Can you work these out from the model? Positions are in its coordinate system, mm. A direction names the side the tool comes from. Coordinates: 2 decimals unless noted, no trailing zeros. Order: outer loops, then holes, each group sorted by start corner. A loop starts at its lowest first (then second) coordinate and runs counter-clockwise, first axis right, second up. Notation, with made-up numbers: (54.5, 28) -> (83.5, 28) arc R33 ccw to (83.5, 60) -> close; hole circle Ø10 at (81, 74). An arc over 180 degrees is marked (long way). Answer in a Markdown table with one row per item.
```python
from build123d import *

# Parameters (mm, degrees)
SKETCH1_W           = 42.3
SKETCH1_H           = 42.3
SKETCH1_R           = 1.75
SKETCH1_R_2         = 11.5
BOSS_EXTRUDE1_DEPTH = 8
BOSS_EXTRUDE2_START = -10
BOSS_EXTRUDE2_DEPTH = 22.3
SKETCH4_R           = 2.75
CUT_EXTRUDE1_DEPTH  = 62.713839627
SKETCH5_R           = 3.75
SKETCH5_R_2         = 1.75
BOSS_EXTRUDE3_DEPTH = 4.3
SKETCH7_R           = 4.25
CUT_EXTRUDE2_DEPTH  = 2
CUT_EXTRUDE3_START  = -2
SKETCH8_R           = 4.25
CUT_EXTRUDE3_DEPTH  = 2


with BuildPart() as part:
    # Sketch1 → Boss-Extrude1 (new body)
    with BuildSketch(Plane(origin=(0, 0, 0), x_dir=(1, 0, 0), z_dir=(0, 1, 0))):
        Rectangle(SKETCH1_W, SKETCH1_H)
        with Locations(Location((-15.5, 15.5, 0), (0, 0, 270))):
            Circle(SKETCH1_R, mode=Mode.SUBTRACT)
        with Locations(Location((15.5, 15.5, 0), (0, 0, 90))):
            Circle(SKETCH1_R, mode=Mode.SUBTRACT)
        with Locations(Location((15.5, -15.5, 0), (0, 0, 270))):
            Circle(SKETCH1_R, mode=Mode.SUBTRACT)
        with Locations(Location((-15.5, -15.5, 0), (0, 0, 90))):
            Circle(SKETCH1_R, mode=Mode.SUBTRACT)
        with Locations(Location((0, 0, 0), (0, 0, 270))):
            Circle(SKETCH1_R_2, mode=Mode.SUBTRACT)
    extrude(amount=BOSS_EXTRUDE1_DEPTH)

    # Sketch3 → Boss-Extrude2 (add)
    with BuildSketch(Plane.XY.offset(21.15).offset(BOSS_EXTRUDE2_START)):
        Polygon((-21.15, 8), (-21.15, 18.080453059), (-15.4, 25.004144271), (-15.4, 45.004144271), (-10.4, 45.004144271), (-10.4, 23.198658368), (-16.15, 16.274967156), (-16.15, 8), align=None)
        Polygon((16.15, 16.274967156), (16.15, 8), (21.15, 8), (21.15, 18.080453059), (15.4, 25.004144271), (15.4, 45.004144271), (10.4, 45.004144271), (10.4, 23.198658368), align=None)
    extrude(amount=-BOSS_EXTRUDE2_DEPTH)

    # Sketch4 → Cut-Extrude1 (cut, through all)
    with BuildSketch(Plane.ZY.offset(15.4)):
        with Locations(Location((-6.081010951, 35.004144271, 0), (0, 0, 270))):
            Circle(SKETCH4_R)
        with Locations(Location((6.081010951, 35.004144271, 0), (0, 0, 270))):
            Circle(SKETCH4_R)
    extrude(amount=-CUT_EXTRUDE1_DEPTH, mode=Mode.SUBTRACT)

    # Sketch5 → Boss-Extrude3 (add)
    # profile 1 of 4: a face of its own
    with BuildSketch(Plane(origin=(0, 8, 0), x_dir=(1, 0, 0), z_dir=(0, 1, 0))):
        with Locations(Location((-15.5, 15.5, 0), (0, 0, 90))):
            Circle(SKETCH5_R)
        with Locations(Location((-15.5, 15.5, 0), (0, 0, 270))):
            Circle(SKETCH5_R_2, mode=Mode.SUBTRACT)
    # profile 2 of 4: a face of its own
    with BuildSketch(Plane(origin=(0, 8, 0), x_dir=(1, 0, 0), z_dir=(0, 1, 0))):
        with Locations(Location((15.5, 15.5, 0), (0, 0, 90))):
            Circle(SKETCH5_R)
        with Locations(Location((15.5, 15.5, 0), (0, 0, 90))):
            Circle(SKETCH5_R_2, mode=Mode.SUBTRACT)
    # profile 3 of 4: a face of its own
    with BuildSketch(Plane(origin=(0, 8, 0), x_dir=(1, 0, 0), z_dir=(0, 1, 0))):
        with Locations(Location((15.5, -15.5, 0), (0, 0, 90))):
            Circle(SKETCH5_R)
        with Locations(Location((15.5, -15.5, 0), (0, 0, 270))):
            Circle(SKETCH5_R_2, mode=Mode.SUBTRACT)
    # profile 4 of 4: a face of its own
    with BuildSketch(Plane(origin=(0, 8, 0), x_dir=(1, 0, 0), z_dir=(0, 1, 0))):
        with Locations(Location((-15.5, -15.5, 0), (0, 0, 90))):
            Circle(SKETCH5_R)
        with Locations(Location((-15.5, -15.5, 0), (0, 0, 90))):
            Circle(SKETCH5_R_2, mode=Mode.SUBTRACT)
    extrude(amount=BOSS_EXTRUDE3_DEPTH)

    # Sketch7 → Cut-Extrude2 (cut)
    with BuildSketch(Plane.ZY.offset(15.4)):
        with Locations((-6.081010951, 35.004144271)):
            Circle(SKETCH7_R)
        with Locations((6.081010951, 35.004144271)):
            Circle(SKETCH7_R)
    extrude(amount=-CUT_EXTRUDE2_DEPTH, mode=Mode.SUBTRACT)

    # Sketch8 → Cut-Extrude3 (cut)
    with BuildSketch(Plane(origin=(15.4, 0, 0), x_dir=(0, 0, -1), z_dir=(1, 0, 0)).offset(CUT_EXTRUDE3_START)):
        with Locations(Location((-6.081010951, 35.004144271, 0), (0, 0, 180))):
            Circle(SKETCH8_R)
        with Locations(Location((6.081010951, 35.004144271, 0), (0, 0, 180))):
            Circle(SKETCH8_R)
    extrude(amount=CUT_EXTRUDE3_DEPTH, mode=Mode.SUBTRACT)


solid = part.part
```
(1) We'd pull the mould along Z, two halves only. Please class faces 6 (the flat face through (0, 4, -21.15)), 7 (the cylindrical face through (-11.921, 32.464, 5.028)), 8 (the flat face through (13.23, 19.79, 0.16)): +Z half, -Z half, draft (parallel to the pull), parting line (faces both ways), or undercut.
Response values:
| item | result |
|---|---|
| face 6 | -Z half |
| face 7 | undercut |
| face 8 | draft |
(2) On a 3-axis mill with a long thin cutter (end or side, diameter ignored), from which of +Z, -Z, +X, -X, +Y, -Y can I reach the whole of each face in a straight line? I mean faces 1 (the cylindrical face through (-14.414, 30.855, 5.16)), 2 (the flat face through (-10, 8, -10)), 3 (the cylindrical face through (9.7, 3.94, 6.18)), 4 (the cylindrical face through (14.39, 30.79, -6.63)), 5 (the flat face through (13, 45.004, 0)). Say none if no direction works.
Response values:
| item | result |
|---|---|
| face 1 | -X |
| face 2 | none |
| face 3 | -Y |
| face 4 | +X |
| face 5 | +Z, -Z, +X, -X, +Y |
(3) Will these pins go through, and if not, where does the flat tip stop? pin 1 Ø5 at (y, z) = (12, 16.5) entering from -X; pin 2 Ø3.5 at (y, z) = (35, -6.08) entering from -X; pin 3 Ø8 at (x, y) = (-7.5, 22.5) entering from -Z; pin 4 Ø6 at (y, z) = (38, -0.5) entering from +X.
Response values:
| item | result |
|---|---|
| pin 1 | x = -19.25 |
| pin 2 | through |
| pin 3 | z = -11.15 |
| pin 4 | x = 15.4 |
(4) I need wall thicknesses on line 1 (X direction, y = 6, z = -15.5); line 2 (Z direction, x = 14, y = 34); line 3 (Y direction, x = 15, z = 5). Which ranges of each line are inside material? Lowest first, please. Write a range as [from, to].
Response values:
| item | result |
|---|---|
| line 1 | [-21.15, -17.25], [-13.75, 13.75], [17.25, 21.15] |
| line 2 | [-11.15, -10.21], [-1.95, 1.95], [10.21, 11.15] |
| line 3 | [0, 8], [17.66, 30.89], [39.11, 45] |
(5) Suppose I cut it at A-A (x = 0). Please give me the cut outline in (y, z).
Response values:
| item | result |
|---|---|
| outline | (0, -21.15) -> (8, -21.15) -> (8, -11.5) -> (0, -11.5) -> close; (0, 11.5) -> (8, 11.5) -> (8, 21.15) -> (0, 21.15) -> close |
(6) Suppose I cut it at B-B (z = 15.5). Please give me the cut outline in (x, y).
Response values:
| item | result |
|---|---|
| outline | (-21.15, 0) -> (-17.25, 0) -> (-17.25, 12.3) -> (-19.25, 12.3) -> (-19.25, 8) -> (-21.15, 8) -> close; (-13.75, 0) -> (13.75, 0) -> (13.75, 12.3) -> (11.75, 12.3) -> (11.75, 8) -> (-11.75, 8) -> (-11.75, 12.3) -> (-13.75, 12.3) -> close; (17.25, 0) -> (21.15, 0) -> (21.15, 8) -> (19.25, 8) -> (19.25, 12.3) -> (17.25, 12.3) -> close |
(7) Suppose I cut it at D-D (y = 26.5). Please give me the cut outline in (x, z), and give its area (3 significant figures).
Response values:
| item | result |
|---|---|
| outline | (-15.4, -11.15) -> (-10.4, -11.15) -> (-10.4, 11.15) -> (-15.4, 11.15) -> close; (10.4, -11.15) -> (15.4, -11.15) -> (15.4, 11.15) -> (10.4, 11.15) -> close |
| area | 223 mm2 |
(8) Suppose I cut it at C-C (y = 10). Count the separate pieces of the cut face and the enclosed holes in it, and give its area (3 significant figures).
Response values:
| item | result |
|---|---|
| separate pieces | 6 |
| enclosed holes | 4 |
| area | 361 mm2 |
